Part model, mm, in its own coordinate system. Face numbers are marked on the shaded views. Give positions to 0.01 mm unless a question says otherwise; leave off trailing zeros. Order: outer loops, then holes, each group sorted by start corner. A loop starts at its lowest first (then second) coordinate and runs counter-clockwise, first axis right, second up. Notation, with made-up numbers: M 3,51.25 L 45,51.25 A14 ccw 45,58.25 Z; hole C 30,7 d6. An arc over 180 degrees is marked long. Answer as a JSON object with one key per item and string values.
from build123d import *

# Parameters (mm, degrees)
BOSS_EXTRU_1_DEPTH      = 7
ESQUISSE2_W             = 17.66012
ESQUISSE2_H             = 22.36185
ENL_V_MAT_EXTRU_1_DEPTH = 5
ESQUISSE5_W             = 2
ESQUISSE5_H             = 21.86
ENL_V_MAT_EXTRU_3_DEPTH = 32.702051256
ESQUISSE6_W             = 3
ESQUISSE6_H             = 1
BOSS_EXTRU_2_DEPTH      = 0.48904
ESQUISSE7_W             = 3
ESQUISSE7_H             = 1
BOSS_EXTRU_3_DEPTH      = 0.48904
ESQUISSE8_W             = 3
ESQUISSE8_H             = 1
BOSS_EXTRU_4_DEPTH      = 0.48904
ESQUISSE9_W             = 3
ESQUISSE9_H             = 1
BOSS_EXTRU_5_DEPTH      = 0.48904
ESQUISSE10_W            = 2
ESQUISSE10_H            = 1
BOSS_EXTRU_6_DEPTH      = 0.48904
ESQUISSE11_W            = 2
ESQUISSE11_H            = 1
BOSS_EXTRU_7_DEPTH      = 0.48904


with BuildPart() as part:
    # Esquisse1 → Boss.-Extru.1 (new body)
    with BuildSketch(Plane(origin=(0, 0, 0), x_dir=(1, 0, 0), z_dir=(0, 1, 0))):
        with BuildLine():
            Line((1, 0), (18.66012, 0))
            ThreePointArc((18.66012, 0), (19.367226781, 0.292893219), (19.66012, 1))
            Line((19.66012, 1), (19.66012, 23.36185))
            ThreePointArc((19.66012, 23.36185), (19.367226781, 24.068956781), (18.66012, 24.36185))
            Line((18.66012, 24.36185), (1, 24.36185))
            ThreePointArc((1, 24.36185), (0.292893219, 24.068956781), (0, 23.36185))
            Line((0, 23.36185), (0, 1))
            ThreePointArc((0, 1), (0.292893219, 0.292893219), (1, 0))
        make_face()
    extrude(amount=BOSS_EXTRU_1_DEPTH)

    # Esquisse2 → Enlèv. mat.-Extru.1 (cut)
    with BuildSketch(Plane(origin=(0, 7, 0), x_dir=(1, 0, 0), z_dir=(0, 1, 0))):
        with Locations((9.83006, 12.180925)):
            Rectangle(ESQUISSE2_W, ESQUISSE2_H)
    extrude(amount=-ENL_V_MAT_EXTRU_1_DEPTH, mode=Mode.SUBTRACT)

    # Esquisse5 → Enlèv. mat.-Extru.3 (cut, through all)
    with BuildSketch(Plane(origin=(0, 2, 0), x_dir=(1, 0, 0), z_dir=(0, 1, 0))):
        with Locations((2.36, 12.18)):
            Rectangle(ESQUISSE5_W, ESQUISSE5_H)
    extrude(amount=-ENL_V_MAT_EXTRU_3_DEPTH, mode=Mode.SUBTRACT)

    # Esquisse6 → Boss.-Extru.2 (add)
    with BuildSketch(Plane.XY.offset(-23.36185)):
        with Locations((16.16012, 5.5)):
            Rectangle(ESQUISSE6_W, ESQUISSE6_H)
    extrude(amount=BOSS_EXTRU_2_DEPTH)

    # Esquisse7 → Boss.-Extru.3 (add)
    with BuildSketch(Plane.ZY.offset(-18.66012)):
        with Locations((-20.86185, 5.5)):
            Rectangle(ESQUISSE7_W, ESQUISSE7_H)
    extrude(amount=BOSS_EXTRU_3_DEPTH)

    # Esquisse8 → Boss.-Extru.4 (add)
    with BuildSketch(Plane(origin=(0, 0, -1), x_dir=(-1, 0, 0), z_dir=(0, 0, -1))):
        with Locations((-16.16012, 5.5)):
            Rectangle(ESQUISSE8_W, ESQUISSE8_H)
    extrude(amount=BOSS_EXTRU_4_DEPTH)

    # Esquisse9 → Boss.-Extru.5 (add)
    with BuildSketch(Plane.ZY.offset(-18.66012)):
        with Locations((-3.5, 5.5)):
            Rectangle(ESQUISSE9_W, ESQUISSE9_H)
    extrude(amount=BOSS_EXTRU_5_DEPTH)

    # Esquisse10 → Boss.-Extru.6 (add)
    with BuildSketch(Plane.XY.offset(-23.36185)):
        with Locations((5, 5.5)):
            Rectangle(ESQUISSE10_W, ESQUISSE10_H)
    extrude(amount=BOSS_EXTRU_6_DEPTH)

    # Esquisse11 → Boss.-Extru.7 (add)
    with BuildSketch(Plane(origin=(0, 0, -1), x_dir=(-1, 0, 0), z_dir=(0, 0, -1))):
        with Locations((-5, 5.5)):
            Rectangle(ESQUISSE11_W, ESQUISSE11_H)
    extrude(amount=BOSS_EXTRU_7_DEPTH)


solid = part.part
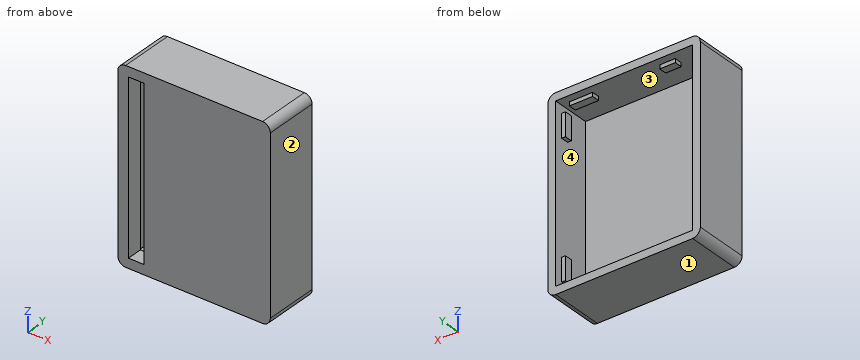
1. Cut at B-B on x = 1.75. Give the cut face in (y, z).
Worked answers:
{"outline": "M 0,-24.36 L 7,-24.36 L 7,-23.36 L 2,-23.36 L 2,-23.11 L 0,-23.11 Z; M 0,-1.25 L 2,-1.25 L 2,-1 L 7,-1 L 7,0 L 0,0 Z"}
2. Probe line 1 along X through (y, z) = (3.5, -22.5); line 2 along Z through (x, y) = (7, 3); line 3 along X through (y, z) = (5.5, -2.5). List the from-to ranges inside material, lowest first.
Worked answers:
{"line 1": "x = 0 to 1, 18.66 to 19.66", "line 2": "z = -24.36 to -23.36, -1 to 0", "line 3": "x = 0 to 1, 18.17 to 19.66"}
3. Two-plate mould, pull along Z, no slides. Class the marked faces 1, 2, 3 and 4: +Z half, -Z half, draft (parallel to the pull), parting line (faces both ways), or undercut.
Worked answers:
{"face 1": "-Z half", "face 2": "draft", "face 3": "undercut", "face 4": "undercut"}
4. Cut at D-D on x = 15.75. Give the cut face in (y, z), plus the area to 3 significant figures.
Worked answers:
{"outline": "M 0,-24.36 L 7,-24.36 L 7,-23.36 L 6,-23.36 L 6,-22.87 L 5,-22.87 L 5,-23.36 L 2,-23.36 L 2,-1 L 5,-1 L 5,-1.49 L 6,-1.49 L 6,-1 L 7,-1 L 7,0 L 0,0 Z", "area": "59.7 mm^2"}
5. Cut at A-A on z = -20.25. Give the cut face in (x, y).
Worked answers:
{"outline": "M 0,0 L 1.36,0 L 1.36,2 L 1,2 L 1,7 L 0,7 Z; M 3.36,0 L 19.66,0 L 19.66,7 L 18.66,7 L 18.66,6 L 18.17,6 L 18.17,5 L 18.66,5 L 18.66,2 L 3.36,2 Z"}
6. Cut at C-C on y = 4.25. Give the cut face in (x, z), plus the area to 3 significant figures.
Worked answers:
{"outline": "M 0,-23.36 A1 ccw 1,-24.36 L 18.66,-24.36 A1 ccw 19.66,-23.36 L 19.66,-1 A1 ccw 18.66,0 L 1,0 A1 ccw 0,-1 Z; hole M 1,-23.36 L 18.66,-23.36 L 18.66,-1 L 1,-1 Z", "area": "83.2 mm^2"}
7. Pin check, flat tips, straight feed: P1, Ø0.5, axis at y = 5.5, z = -3, coming from the -X side; P2, Ø9, axis at x = 10, z = -15.5, coming from the +Y side. Stop position of each tip, or through.
Worked answers:
{"P1": "stops at x = 0", "P2": "stops at y = 2"}
